Geometry check sheet. Reference: the model listing, model coordinates, mm. Give positions to 0.01 mm unless a question says otherwise; leave off trailing zeros. Order: outer loops, then holes, each group sorted by start corner. A loop starts at its lowest first (then second) coordinate and runs counter-clockwise, first axis right, second up.
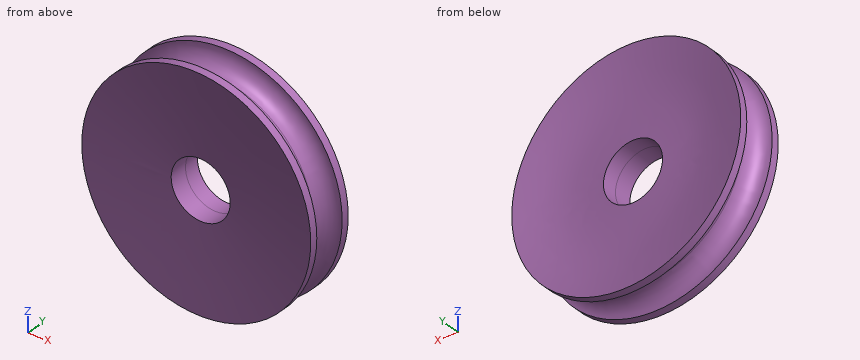
from build123d import *

# Parameters (mm, degrees)
F2_R          = 1
F3_DEPTH      = 9
F3_DEPTH_BACK = 10.2


with BuildPart() as f1:
    # F0 (on Top) → F1 (revolve)
    with BuildSketch(Plane.XY):
        with BuildLine():
            ThreePointArc((-3.3291771512, 0), (-3.4902684216, -0.3889087297), (-3.8791771512, -0.55))
            Line((-3.8791771512, -0.55), (-3.8791771512, -0.8130174247))
            add(Edge.make_bspline(
                [(-3.8791771512, -0.8130174247), (-3.3627895766, -0.7711625564), (-2.2360945011, -0.6798403088), (-0.7856667947, -0.6088802847), (0, -0.5704427022)],
                knots=[0, 0, 0, 0, 0.4583206103, 1, 1, 1, 1], degree=3))
            Line((0, -0.5704427022), (0, 0))
            Line((0, 0), (0, 0.55))
            add(Edge.make_bspline(
                [(-3.8791771512, 0.813), (-3.3637205638, 0.7051800282), (-2.2426051819, 0.4706721533), (-0.7865843545, 0.5221760908), (0, 0.55)],
                knots=[0, 0, 0, 0, 0.4597712206, 1, 1, 1, 1], degree=3))
            Line((-3.8791771512, 0.813), (-3.8791771512, 0.55))
            ThreePointArc((-3.8791771512, 0.55), (-3.4902684216, 0.3889087297), (-3.3291771512, 0))
        make_face()
    revolve(axis=Axis((0, 0.275, 0), (0, 1, 0)))

    # F2 (on Front) → F3 (cut, two sides)
    with BuildSketch(Plane.XZ) as f3_sk:
        Circle(F2_R)
    extrude(amount=-F3_DEPTH, mode=Mode.SUBTRACT)
    extrude(f3_sk.sketch, amount=F3_DEPTH_BACK, mode=Mode.SUBTRACT)


solid = f1.part
Item 1: Scan lines: L1, parallel to Z at x = 0.5, y = -0.2; L2, parallel to Z at x = 0, y = 0.45; L3, parallel to X at y = -0.2, z = 0.25. Record each from-to range of solid material in increasing order.
Reported:
L1: z = -3.33 to -0.87, 0.87 to 3.33
L2: z = -3.56 to -1, 1 to 3.56
L3: x = -3.36 to -0.97, 0.97 to 3.36
Item 2: Sectioned sample at A-A (y = 0.15). Enter the section's corners in (x, z), and give its area (3 significant figures).
Reported:
outline: circle Ø6.7 at (0, 0); hole circle Ø2 at (0, 0)
area: 32.1 mm2
Item 3: Gauge pin test, flat end, axial feed: pin 1 (2.5 mm diameter, centred on x = 0, z = 0, fed in from +Y). Record the tip position at first contact, or that the pin passes through.
Reported:
pin 1: stops at y = 0.52
